from build123d import *

# Parameters (mm, degrees)
SKETCH1_W           = 177.8
SKETCH1_H           = 63.5
SKETCH1_R           = 2.032
BOSS_EXTRUDE1_DEPTH = 6.35
SKETCH2_R           = 2.413
CUT_EXTRUDE1_DEPTH  = 6.35
LPATTERN1_COUNT     = 3
LPATTERN1_PITCH     = 12.7


with BuildPart() as part:
    # Sketch1 → Boss-Extrude1 (new body)
    with BuildSketch(Plane.XY):
        Rectangle(SKETCH1_W, SKETCH1_H)
        with Locations((-82.804, 25.654)):
            Circle(SKETCH1_R, mode=Mode.SUBTRACT)
        with Locations((-82.804, 0)):
            Circle(SKETCH1_R, mode=Mode.SUBTRACT)
        with Locations((-82.804, -25.654)):
            Circle(SKETCH1_R, mode=Mode.SUBTRACT)
        with Locations((82.804, -25.654)):
            Circle(SKETCH1_R, mode=Mode.SUBTRACT)
        with Locations((82.804, 0)):
            Circle(SKETCH1_R, mode=Mode.SUBTRACT)
        with Locations((82.804, 25.654)):
            Circle(SKETCH1_R, mode=Mode.SUBTRACT)
    extrude(amount=BOSS_EXTRUDE1_DEPTH)

    # Sketch2 → Cut-Extrude1 (cut)
    with BuildSketch(Plane.XY.offset(6.35)):
        with Locations((63.5, 19.05)):
            Circle(SKETCH2_R)
    cut_extrude1 = extrude(amount=-CUT_EXTRUDE1_DEPTH, mode=Mode.SUBTRACT)

    # LPattern1: Cut-Extrude1 ×3
    with Locations(*[(0, -i * LPATTERN1_PITCH, 0) for i in range(1, LPATTERN1_COUNT)]):
        add(cut_extrude1, mode=Mode.SUBTRACT)


solid = part.part
For this review, take the finished solid that the model builds, in its own axes (mm). Coordinates: 2 decimals unless noted, no trailing zeros. Loops run counter-clockwise (first coordinate to the right, second up) from the corner with the lowest first, then second, coordinate; pieces in that order, holes last. Notation, with made-up numbers: (49.5, -33.5) - (60.5, -33.5) arc R12 cw to (60.5, -25.5) - close; hole circle Ø5 at (89, -35). An arc over 180 degrees is marked (long way). Return JSON: item names as keys, results as strings.
Item 1: Mouldability with a two-part tool opening along X and no side actions: class faces 1 (the flat face through (-88.9, 0, 3)), 2 (the cylindrical face through (84.68, -0.78, 3.13)), 3 (the flat face through (-1, -31.75, 3)) as pulls with the +X half, pulls with the -X half, needs draft (parallel to the pull), parting line crosses it, or undercut.
Determined:
{"face 1": "pulls with the -X half", "face 2": "undercut", "face 3": "needs draft"}
Item 2: Insertion check: pin 1 (6.5 mm diameter, centred on x = 63.5, y = -6.35, fed in from +Z). The pin has a flat end and moves straight along its axis. Give the tip position at first contact, or say it passes through.
Determined:
{"pin 1": "stops at z = 6.35"}
Item 3: For line 1 (X direction, y = -26, z = 1.25); line 2 (Y direction, x = 63.5, z = 2.75); line 3 (X direction, y = 6, z = 4.75), list the stretches that pass through material, from the lowest coordinate up.
Determined:
{"line 1": "x = -88.9 to -84.81, -80.8 to 80.8, 84.81 to 88.9", "line 2": "y = -31.75 to -8.76, -3.94 to 3.94, 8.76 to 16.64, 21.46 to 31.75", "line 3": "x = -88.9 to 61.11, 65.89 to 88.9"}
Item 4: Take a section at B-B (x = 63.5). Give the boundary of the cut face in (y, z).
Determined:
{"outline": "(-31.75, 0) - (-8.76, 0) - (-8.76, 6.35) - (-31.75, 6.35) - close; (-3.94, 0) - (3.94, 0) - (3.94, 6.35) - (-3.94, 6.35) - close; (8.76, 0) - (16.64, 0) - (16.64, 6.35) - (8.76, 6.35) - close; (21.46, 0) - (31.75, 0) - (31.75, 6.35) - (21.46, 6.35) - close"}
Item 5: Take a section at A-A (y = -6.35). Give the boundary of the cut face in (x, z).
Determined:
{"outline": "(-88.9, 0) - (61.09, 0) - (61.09, 6.35) - (-88.9, 6.35) - close; (65.91, 0) - (88.9, 0) - (88.9, 6.35) - (65.91, 6.35) - close"}
